from build123d import *

# Parameters (mm, degrees)
SKETCH_1_R      = 4.5
SKETCH_1_R_2    = 2
EXTRUDE_1_DEPTH = 5


with BuildPart() as part:
    # 草图1 → 凸台-拉伸1 (new body)
    with BuildSketch(Plane(origin=(0, 0, 0), x_dir=(1, 0, 0), z_dir=(0, 1, 0))):
        with BuildLine():
            Line((-140.609734673, 23.423817863), (73.390265327, 23.423817863))
            ThreePointArc((73.390265327, 23.423817863), (82.390265327, 14.423817863), (73.390265327, 5.423817863))
            Line((73.390265327, 5.423817863), (-140.609734673, 5.423817863))
            ThreePointArc((-140.609734673, 5.423817863), (-149.609734673, 14.423817863), (-140.609734673, 23.423817863))
        make_face()
        with Locations(Location((-140.609734673, 14.423817863, 0), (0, 0, 270))):
            Circle(SKETCH_1_R, mode=Mode.SUBTRACT)
        with Locations(Location((73.390265327, 14.423817863, 0), (0, 0, 270))):
            Circle(SKETCH_1_R, mode=Mode.SUBTRACT)
        with Locations(Location((38.390265327, 14.423817863, 0), (0, 0, 270))):
            Circle(SKETCH_1_R_2, mode=Mode.SUBTRACT)
        with Locations(Location((19.390265327, 14.423817863, 0), (0, 0, 270))):
            Circle(SKETCH_1_R, mode=Mode.SUBTRACT)
        with Locations(Location((-105.609734673, 14.423817863, 0), (0, 0, 270))):
            Circle(SKETCH_1_R_2, mode=Mode.SUBTRACT)
    extrude(amount=EXTRUDE_1_DEPTH)


solid = part.part
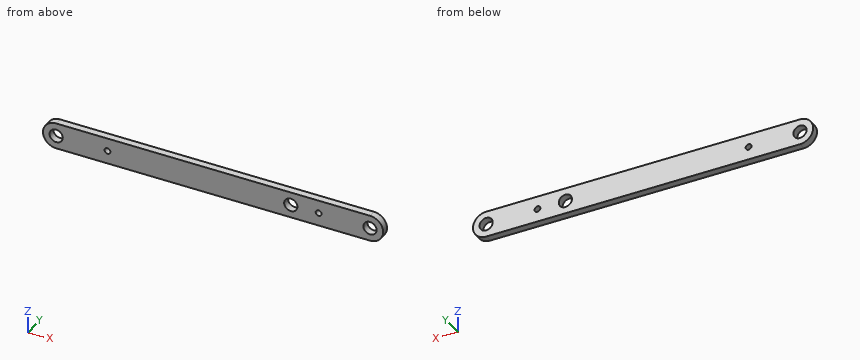
Work out the finished part from the listing and answer in its coordinate system (mm). Round coordinates to 2 decimals unless told otherwise and drop trailing zeros. Write each loop counter-clockwise with the first axis right and the second up, starting at its lowest first coordinate (ties: lowest second). Pieces come first, ordered by that corner, then holes.
1) A cutting plane is placed at A-A (y = 3.4). Give the vertices of the cut face in (x, z).
2) Given pin 1 Ø3.5 at (x, z) = (-105.61, -14.42) entering from -Y, flat-ended and moving along its own axis, determine where the tip first touches the part or whether it passes through.
3) Straight lines are drawn through the part: line 1 (X direction, y = 2.75, z = -16.5); line 2 (X direction, y = 4.7, z = -16); line 3 (X direction, y = 0.85, z = -11.75). For each, find the intervals that lie inside material, in ascending order.
Completed:
1. outline: (-140.61, -23.42) - (73.39, -23.42) arc R9 ccw to (73.39, -5.42) - (-140.61, -5.42) arc R9 ccw to start; hole circle Ø9 at (-140.61, -14.42); hole circle Ø4 at (-105.61, -14.42); hole circle Ø9 at (19.39, -14.42); hole circle Ø4 at (38.39, -14.42); hole circle Ø9 at (73.39, -14.42)
2. pin 1: passes through
3. line 1: x = -149.37 to -144.6, -136.62 to 15.4, 23.38 to 69.4, 77.38 to 82.15
3. line 2: x = -149.47 to -144.82, -136.39 to -106.84, -104.38 to 15.18, 23.61 to 37.16, 39.62 to 69.18, 77.61 to 82.25
3. line 3: x = -149.2 to -144.23, -136.99 to 15.77, 23.01 to 69.77, 77.01 to 81.98
